Check sheet for the modelled part. Datum: model origin and axes. Units: mm. Face numbers are marked on the shaded views. A direction names the side the tool comes from. Coordinates: 2 decimals unless noted, no trailing zeros. Write each loop counter-clockwise with the first axis right and the second up, starting at its lowest first coordinate (ties: lowest second). Pieces come first, ordered by that corner, then holes. Notation, with made-up numbers: (1, 30.5) - (10, 30.5) arc R27 cw to (10, 60.5) - close; hole circle Ø6 at (67, -37.75). An arc over 180 degrees is marked (long way). Use one line per item in the form item = value. Start each with the question number.
1. Tool access check on the marked faces 1 and 2. Record the directions out of +Z, -Z, +X, -X, +Y, -Y that give a thin tool (end or side, any length) a straight path to the whole face; none if there is none.
2. Cross-section at D-D on y = 5. Record the boundary of the cut face in (x, z).
3. Cross-section at A-A on z = 6. Record the boundary of the cut face in (x, y).
4. Cross-section at C-C on x = 5. Record the boundary of the cut face in (y, z), then the cut area to 3 significant figures.
5. Scan lines: line 1 along Y through (x, z) = (0, 22.25); line 2 along Y through (x, z) = (0, -15); line 3 along X through (y, z) = (0, 21.75). Record each from-to range of solid material in increasing order.
6. Go/stop test with flat-tipped pins: pin 1 Ø4 at (x, z) = (-2.5, -16.5) entering from +Y; pin 2 Ø2.5 at (x, y) = (0, 0) entering from -Z; pin 3 Ø3 at (x, y) = (0, 0) entering from +Z. Record where each tip stops, or that it passes through.
7. Cross-section at B-B on z = -22. Record the boundary of the cut face in (x, y).
```python
from build123d import *

# Parameters (mm, degrees)
BASE_EXTRUSION_DEPTH = 28
ESQUISSE2_R          = 4
BOSS_EXTRU_1_DEPTH   = 38.5
PER_AGE1_D           = 3.3
PER_AGE1_DEPTH       = 25
PER_AGE1_TIP         = 0.991420021
PER_AGE2_D           = 3.3
PER_AGE2_DEPTH       = 25
PER_AGE2_TIP         = 0.991420021


with BuildPart() as part:
    # Esquisse1 → Base-Extrusion (new body)
    with BuildSketch(Plane.XY):
        Polygon((0, 6.92820323), (-6, 3.464101615), (-6, -3.464101615), (0, -6.92820323), (6, -3.464101615), (6, 3.464101615), align=None)
    extrude(amount=BASE_EXTRUSION_DEPTH)

    # Esquisse2 → Boss.-Extru.1 (add)
    with BuildSketch(Plane(origin=(0, 0, 0), x_dir=(-1, 0, 0), z_dir=(0, 0, -1))):
        with Locations(Location((0, 0, 0), (0, 0, 180))):
            Circle(ESQUISSE2_R)
    extrude(amount=BOSS_EXTRU_1_DEPTH)

    # Perçage1
    with Locations(Plane.XY.offset(28)):
        with Locations((0, 0)):
            Hole(PER_AGE1_D / 2, depth=PER_AGE1_DEPTH)
            with Locations((0, 0, -(PER_AGE1_DEPTH + PER_AGE1_TIP / 2))):  # 118° drill point
                Cone(0, PER_AGE1_D / 2, PER_AGE1_TIP, mode=Mode.SUBTRACT)

    # Perçage2
    with Locations(Plane(origin=(0, 0, -38.5), x_dir=(-1, 0, 0), z_dir=(0, 0, -1))):
        with Locations((0, 0)):
            Hole(PER_AGE2_D / 2, depth=PER_AGE2_DEPTH)
            with Locations((0, 0, -(PER_AGE2_DEPTH + PER_AGE2_TIP / 2))):  # 118° drill point
                Cone(0, PER_AGE2_D / 2, PER_AGE2_TIP, mode=Mode.SUBTRACT)


solid = part.part
```
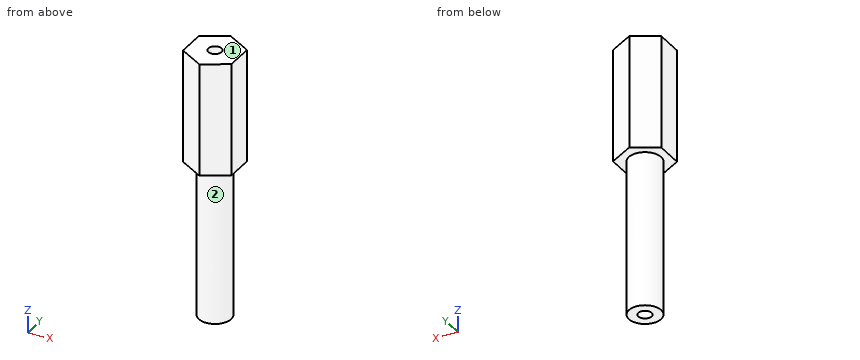
Final values:
q1.face_1 = +Z, +X, -X, +Y, -Y
q1.face_2 = -Z
q2.outline = (-3.34, 0) - (3.34, 0) - (3.34, 28) - (-3.34, 28) - close
q3.outline = (-6, -3.46) - (0, -6.93) - (6, -3.46) - (6, 3.46) - (0, 6.93) - (-6, 3.46) - close; hole circle Ø3.3 at (0, 0)
q4.outline = (-4.04, 0) - (4.04, 0) - (4.04, 28) - (-4.04, 28) - close
q4.area = 226 mm²
q5.line_1 = -6.93 to -1.65, 1.65 to 6.93
q5.line_2 = -4 to -1.65, 1.65 to 4
q5.line_3 = -6 to -1.65, 1.65 to 6
q6.pin_1 = 3.97
q6.pin_2 = -13.26
q6.pin_3 = 2.91
q7.outline = circle Ø8 at (0, 0); hole circle Ø3.3 at (0, 0)
